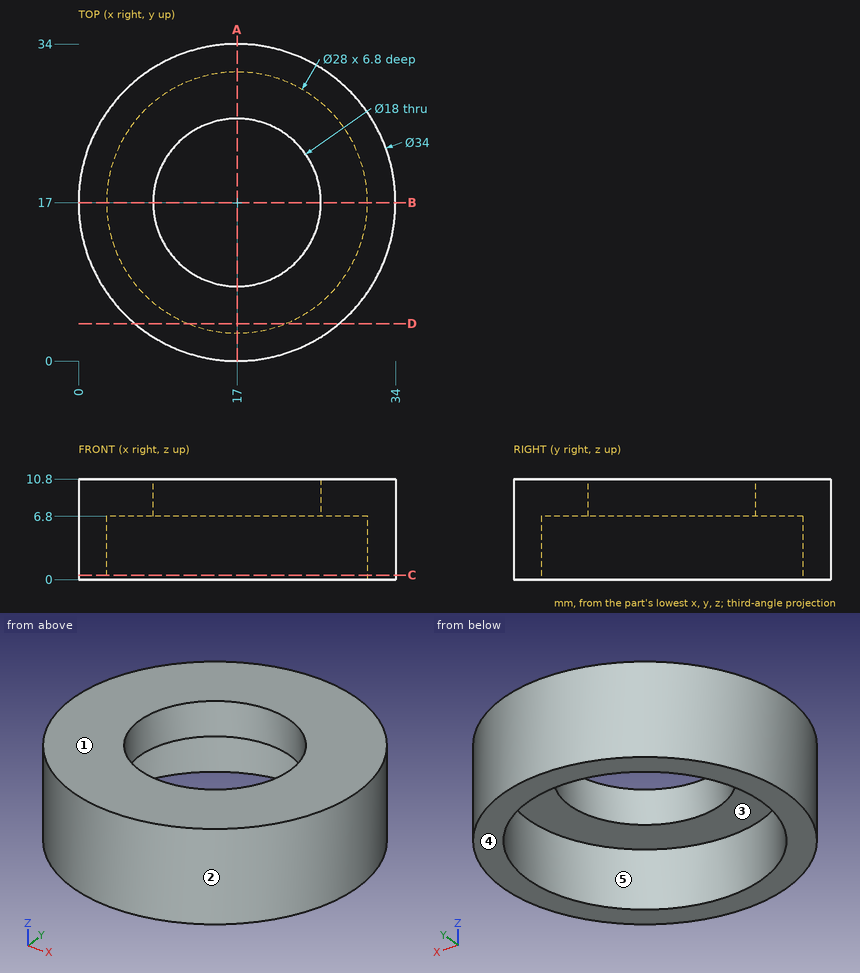
Study the drawing (mm; zero at the part's minimum x, y, z) and answer. A direction names the side the tool comes from. Give positions to 0.01 mm unless a question says otherwise; leave off trailing zeros. Order: outer loops, then holes, each group sorted by start corner. A loop starts at its lowest first (then second) coordinate and runs counter-clockwise, first axis right, second up. Notation, with made-up numbers: (64.5, 26) - (96.5, 26) arc R16 ccw to (96.5, 50) - close; hole circle Ø10 at (21, 42). An arc over 180 degrees is marked (long way). Answer as CSV lines item,"result". Start each with the question number.
Q1. The part is cut by section A-A (x = 17). Write down the section's boundary in (y, z), then the cut area to 3 significant figures.
Q2. The part is cut by section D-D (y = 4). Write down the section's boundary in (x, z), then the cut area to 3 significant figures.
Q3. For the marked faces 4 and 5, determine the directions among +Z, -Z, +X, -X, +Y, -Y from which every point of the face is accessible in a straight line to the end or side of a thin tool.
Q4. The mould has two halves that part along X. Classify the marked faces 1, 2 and 3: +X half, -X half, draft (parallel to the pull), parting line (faces both ways), or undercut.
Q5. Find the intervals of material crossed by L1, parallel to Y at x = 17, z = 9.1; L2, parallel to Y at x = 19, z = 3; L3, parallel to X at y = 22.5, z = 10.25, in increasing order. Write a range as [from, to].
Q6. The part is cut by section C-C (z = 0.5). Write down the section's boundary in (x, y), then the cut area to 3 significant figures.
Q7. Given pin 1 Ø5 at (y, z) = (24, 5) entering from -X; pin 2 Ø3 at (x, z) = (13.5, 5.5) entering from -Y; pin 3 Ø8 at (x, y) = (12, 22) entering from -Z, each flat-ended and moving along its own axis, determine where each tip first touches the part or whether it passes through.
Check result:
1,outline,"(0, 0) - (3, 0) - (3, 6.8) - (8, 6.8) - (8, 10.8) - (0, 10.8) - close; (26, 6.8) - (31, 6.8) - (31, 0) - (34, 0) - (34, 10.8) - (26, 10.8) - close"
1,area,"105 mm²"
2,outline,"(6.05, 0) - (11.8, 0) - (11.8, 6.8) - (22.2, 6.8) - (22.2, 0) - (27.95, 0) - (27.95, 10.8) - (6.05, 10.8) - close"
2,area,"166 mm²"
3,face 4,"-Z, +X, -X, +Y, -Y"
3,face 5,"-Z"
4,face 1,"draft"
4,face 2,"parting line"
4,face 3,"undercut"
5,L1,"y = [0, 8], [26, 34]"
5,L2,"y = [0.12, 3.14], [30.86, 33.88]"
5,L3,"x = [0.91, 9.88], [24.12, 33.09]"
6,outline,"circle Ø34 at (17, 17); hole circle Ø28 at (17, 17)"
6,area,"292 mm²"
7,pin 1,"stops at x = 0.61"
7,pin 2,"stops at y = 0.12"
7,pin 3,"stops at z = 6.8"
